Read the model definition and answer for the solid it produces. Units are mm, in the model's axes. Coordinates: 2 decimals unless noted, no trailing zeros. Loops run counter-clockwise (first coordinate to the right, second up) from the corner with the lowest first, then second, coordinate; pieces in that order, holes last. Notation, with made-up numbers: M 58,15.5 L 66,15.5 A8 ccw 66,26.5 Z; hole C 46,-3 d8. An arc over 180 degrees is marked long. Use one line per item in the form item = value. Start each with the question number.
1. Find the intervals of material crossed by probe 1 along X at (y, z) = (23.5, 2.2); probe 2 along X at (y, z) = (56.5, 2.35); probe 3 along X at (y, z) = (34.5, 1.8), in increasing order. Write a range as [from, to].
2. The part is cut by section B-B (y = 22). Give the vertices of the cut face in (x, z) (3 decimals), plus the area to 3 significant figures.
3. The part is cut by section D-D (y = 11). Give the vertices of the cut face in (x, z).
4. Flat-ended cylindrical pins translate along their axes: pin 1 (1.5 mm diameter, centred on y = 19.5, z = 0.5, fed in from +X); pin 2 (1 mm diameter, centred on y = 51.5, z = 2, fed in from -X). Find the tip coordinate at first contact, or state that the pin passes through.
5. The part is cut by section A-A (z = 1.25). Give the vertices of the cut face in (x, y).
6. The part is cut by section C-C (x = 61.5). Give the vertices of the cut face in (y, z).
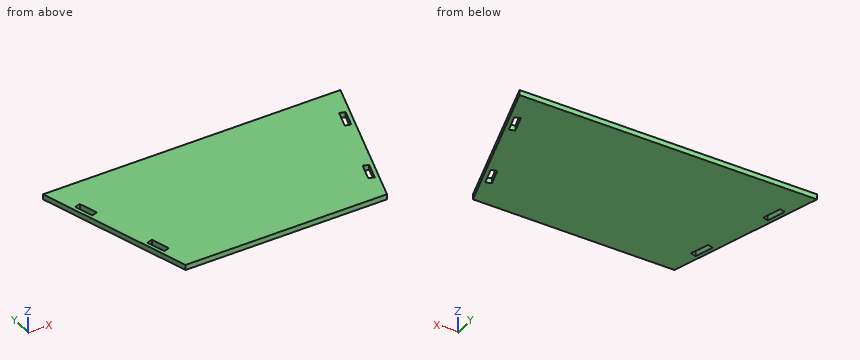
from build123d import *

# Parameters (mm, degrees)
BOSS_EXTRUDE1_DEPTH = 2.75
CUT_EXTRUDE1_DEPTH  = 10


with BuildPart() as part:
    # Sketch1 → Boss-Extrude1 (new body)
    with BuildSketch(Plane.XY):
        Polygon((-52.5, 0), (52.5, 0), (77.5, 80), (-77.5, 80), align=None)
    extrude(amount=BOSS_EXTRUDE1_DEPTH)

    # Sketch4 → Cut-Extrude1 (cut)
    with BuildSketch(Plane.XY.offset(2.75)):
        Polygon((70.437485367, 64.105175021), (67.454735436, 54.56037524), (64.591295502, 55.45520022), (67.574045433, 65), align=None)
        Polygon((57.795235299, 23.649974801), (54.812485367, 14.105175021), (51.949045433, 15), (54.931795364, 24.54479978), align=None)
        Polygon((-54.931795364, 24.54479978), (-51.949045433, 15), (-54.812485367, 14.105175021), (-57.795235299, 23.649974801), align=None)
        Polygon((-67.574045433, 65), (-64.591295502, 55.45520022), (-67.454735436, 54.56037524), (-70.437485367, 64.105175021), align=None)
    extrude(amount=-CUT_EXTRUDE1_DEPTH, mode=Mode.SUBTRACT)


solid = part.part
Computed values:
q1.probe_1 = [-59.84, -57.75], [-54.61, 54.61], [57.75, 59.84]
q1.probe_2 = [-70.16, -68.06], [-64.92, 64.92], [68.06, 70.16]
q1.probe_3 = [-63.28, 63.28]
q2.outline = M -59.375,0 L -57.28,0 L -57.28,2.75 L -59.375,2.75 Z; M -54.137,0 L 54.137,0 L 54.137,2.75 L -54.137,2.75 Z; M 57.28,0 L 59.375,0 L 59.375,2.75 L 57.28,2.75 Z
q2.area = 309 mm²
q3.outline = M -55.94,0 L 55.94,0 L 55.94,2.75 L -55.94,2.75 Z
q4.pin_1 = 58.83
q4.pin_2 = -68.75
q5.outline = M -77.5,80 L -52.5,0 L 52.5,0 L 77.5,80 Z; hole M -70.44,64.11 L -67.45,54.56 L -64.59,55.46 L -67.57,65 Z; hole M -57.8,23.65 L -54.81,14.11 L -51.95,15 L -54.93,24.54 Z; hole M 51.95,15 L 54.81,14.11 L 57.8,23.65 L 54.93,24.54 Z; hole M 64.59,55.46 L 67.45,54.56 L 70.44,64.11 L 67.57,65 Z
q6.outline = M 28.8,0 L 80,0 L 80,2.75 L 28.8,2.75 Z
